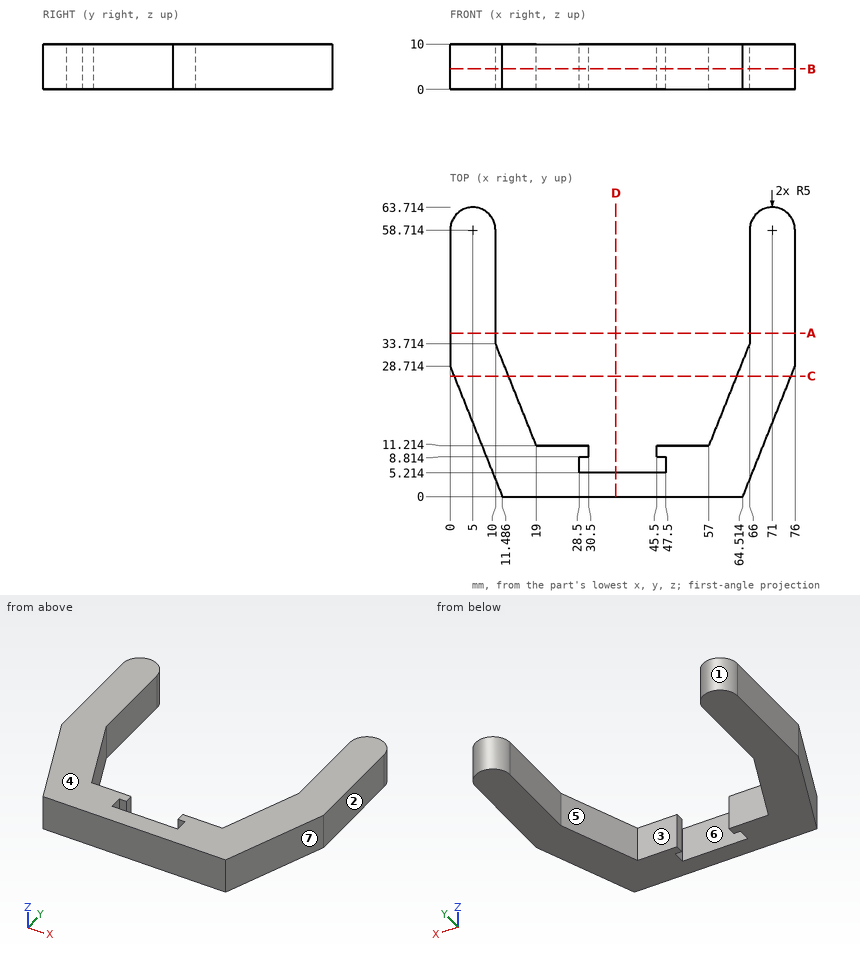
Job drawing, mm, ordinate dimensions from the low corner. One solid piece. A direction names the side the tool comes from. Give positions to 0.01 mm unless a question says otherwise; leave off trailing zeros. Order: outer loops, then holes, each group sorted by start corner. A loop starts at its lowest first (then second) coordinate and runs counter-clockwise, first axis right, second up. Notation, with made-up numbers: (55.25, 69) - (93.25, 69) arc R16 cw to (93.25, 91) - close; hole circle Ø10 at (51, 72.5). An arc over 180 degrees is marked (long way). Return JSON: item names as keys, results as strings.
1) Cut at C-C, the plane y = 26.5. Give the cut face in (x, z) (1 decimal), plus the area to 3 significant figures.
Geometry says:
{"outline": "(0.9, 0) - (12.9, 0) - (12.9, 10) - (0.9, 10) - close; (63.1, 0) - (75.1, 0) - (75.1, 10) - (63.1, 10) - close", "area": "240 mm²"}
2) Cut at D-D, the plane x = 36.5. Give the cut face in (y, z).
Geometry says:
{"outline": "(0, 0) - (5.21, 0) - (5.21, 10) - (0, 10) - close"}
3) Probe line 1 (X direction, y = 59, z = 1.75); line 2 (X direction, y = 32.5, z = 0.5) (1 decimal); line 3 (Y direction, x = 31, z = 1.5). List the from-to ranges inside material, lowest first. Write a range as from..to.
Geometry says:
{"line 1": "0.01..9.99, 66.01..75.99", "line 2": "0..10.5, 65.5..76", "line 3": "0..5.21"}
4) 3-axis set-ups, long thin cutter, end or side, ignore diameter. For the marked faces 5, 6 and 7: which of +Z, -Z, +X, -X, +Y, -Y reach the whole face in a straight line?
Geometry says:
{"face 5": "+Z, -Z, +Y", "face 6": "+Z, -Z", "face 7": "+Z, -Z, +X, -Y"}
5) Pull direction X, two halves, no side cores. Call the marked faces 1, 2, 3 and 4: pulls with the +X half, pulls with the -X half, needs draft (parallel to the pull), parting line crosses it, or undercut.
Geometry says:
{"face 1": "undercut", "face 2": "pulls with the +X half", "face 3": "undercut", "face 4": "needs draft"}
6) Cut at A-A, the plane y = 36. Give the cut face in (x, z).
Geometry says:
{"outline": "(0, 0) - (10, 0) - (10, 10) - (0, 10) - close; (66, 0) - (76, 0) - (76, 10) - (66, 10) - close"}
7) Flat gauge pins, fed straight in: P1, Ø1.9, axis at y = 10.5, z = 4.5, coming from the +X side (1 decimal); P2, Ø0.7, axis at y = 10, z = 5.5, coming from the -X side (1 decimal); P3, Ø1, axis at x = 66, z = 8, coming from the +Y side (1 decimal). Where does each tip first touch, or does it go through?
Geometry says:
{"P1": "x = 69.1", "P2": "x = 7.3", "P3": "y = 60.9"}
8) Cut at B-B, the plane z = 4.5. Give the cut face in (x, y) (1 decimal), plus the area to 3 significant figures.
Geometry says:
{"outline": "(0, 28.7) - (11.5, 0) - (64.5, 0) - (76, 28.7) - (76, 58.7) arc R5 ccw to (66, 58.7) - (66, 33.7) - (57, 11.2) - (45.5, 11.2) - (45.5, 8.8) - (47.5, 8.8) - (47.5, 5.2) - (28.5, 5.2) - (28.5, 8.8) - (30.5, 8.8) - (30.5, 11.2) - (19, 11.2) - (10, 33.7) - (10, 58.7) arc R5 ccw to (0, 58.7) - close", "area": "1,650 mm²"}
